Geometry check sheet. Reference: the model listing, model coordinates, mm. A direction names the side the tool comes from. Round coordinates to 2 decimals unless told otherwise and drop trailing zeros. Loops run counter-clockwise (first coordinate to the right, second up) from the corner with the lowest first, then second, coordinate; pieces in that order, holes last.
```python
from build123d import *

# Parameters (mm, degrees)
F0_R            = 6.35
F1_DEPTH        = 9.525
F2_W            = 9.5377
F2_H            = 31.75
F3_DEPTH        = 1.5875
F5_D            = 5.159375
F5_DEPTH        = 19.05
F5_TIP          = 1.5500326281
F7_D            = 3.571875
F7_DEPTH        = 19.05
F7_TIP          = 1.0730995118
F10_D           = 3.571875
F10_DEPTH       = 12.7
F10_TIP         = 1.0730995118
F10_ON_F9_D     = 3.571875
F10_ON_F9_DEPTH = 12.7
F10_ON_F9_TIP   = 1.0730995118


with BuildPart() as f1:
    # F0 (on Front) → F1 (new body)
    with BuildSketch(Plane.XZ):
        with BuildLine():
            Line((0, 50.8), (0, 0))
            Line((0, 0), (298.45, 0))
            Line((298.45, 0), (298.45, 50.8))
            Line((298.45, 50.8), (111.1377, 50.8))
            Line((111.1377, 50.8), (111.1377, 38.1))
            ThreePointArc((111.1377, 38.1), (114.3127, 34.925), (111.1377, 31.75))
            Line((111.1377, 31.75), (101.6, 31.75))
            ThreePointArc((101.6, 31.75), (98.425, 34.925), (101.6, 38.1))
            Line((101.6, 38.1), (101.6, 50.8))
            Line((101.6, 50.8), (88.9, 50.8))
            Line((88.9, 50.8), (88.9, 23.8125))
            ThreePointArc((88.9, 23.8125), (82.55, 17.4625), (76.2, 23.8125))
            Line((76.2, 23.8125), (76.2, 50.8))
            Line((76.2, 50.8), (0, 50.8))
        make_face()
        with Locations((250.19, 25.4)):
            Circle(F0_R, mode=Mode.SUBTRACT)
    extrude(amount=F1_DEPTH)

    # F2 (on face) → F3 (cut)
    with BuildSketch(Plane.XZ.offset(9.525)):
        with Locations((106.36885, 15.875)):
            Rectangle(F2_W, F2_H)
    extrude(amount=-F3_DEPTH, mode=Mode.SUBTRACT)

    # F5
    with Locations(Plane(origin=(0, 0, 0), x_dir=(0, -1, 0), z_dir=(-1, 0, 0))):
        with Locations((4.7625, 38.1), (4.7625, 25.4), (4.7625, 12.7)):
            Hole(F5_D / 2, depth=F5_DEPTH)
            with Locations((0, 0, -(F5_DEPTH + F5_TIP / 2))):  # 118° drill point
                Cone(0, F5_D / 2, F5_TIP, mode=Mode.SUBTRACT)

    # F7
    with Locations(Plane.XY.offset(31.75)):
        with Locations((106.36885, -3.96875)):
            Hole(F7_D / 2, depth=F7_DEPTH)
            with Locations((0, 0, -(F7_DEPTH + F7_TIP / 2))):  # 118° drill point
                Cone(0, F7_D / 2, F7_TIP, mode=Mode.SUBTRACT)

    # F10
    with Locations(Plane.XY.offset(50.8)):
        with Locations((38.1, -4.7625), (260.35, -4.7625)):
            Hole(F10_D / 2, depth=F10_DEPTH)
            with Locations((0, 0, -(F10_DEPTH + F10_TIP / 2))):  # 118° drill point
                Cone(0, F10_D / 2, F10_TIP, mode=Mode.SUBTRACT)

    # F10 on F9
    with Locations(Plane(origin=(0, 0, 0), x_dir=(1, 0, 0), z_dir=(0, 0, -1))):
        with Locations((260.35, 4.7625), (38.1, 4.7625)):
            Hole(F10_ON_F9_D / 2, depth=F10_ON_F9_DEPTH)
            with Locations((0, 0, -(F10_ON_F9_DEPTH + F10_ON_F9_TIP / 2))):  # 118° drill point
                Cone(0, F10_ON_F9_D / 2, F10_ON_F9_TIP, mode=Mode.SUBTRACT)


solid = f1.part
```
1) Mould release check, pull along Z, two halves, no side actions. Record for faces 1 (the face through (101.6, -5, 44)), 2 (the face through (39, -7, 50.8)), 3 (the face through (256.056, -4.696, 22.968)): +Z half, -Z half, draft (parallel to the pull), parting line (faces both ways), or undercut.
Report:
face 1: draft
face 2: +Z half
face 3: undercut
2) Scan lines: line 1 along X through (y, z) = (-7, 46); line 2 along Y through (x, z) = (260.35, 48) (3 decimals); line 3 along X through (y, z) = (-6, 21). Record each from-to range of solid material in increasing order.
Report:
line 1: x = 0 to 76.2, 88.9 to 101.6, 111.14 to 298.45
line 2: y = -9.525 to -6.548, -2.977 to 0
line 3: x = 0 to 76.86, 88.24 to 245.61, 254.77 to 298.45
3) Sectioned sample at B-B, the plane x = 82.55. Record the cut outline in (y, z) (1 decimal).
Report:
outline: (-9.5, 0) - (0, 0) - (0, 17.5) - (-9.5, 17.5) - close
4) Access from +Z, -Z, +X, -X, +Y, -Y to the whole of each face (thin tool, end or side, straight path). Record for faces 4 (the face through (9.658, -5.098, 40.658)), 5 (the face through (98.426, -4.696, 34.855)), 6 (the face through (88.9, -5, 37)).
Report:
face 4: -X
face 5: +Y, -Y
face 6: +Z, +Y, -Y
5) Sectioned sample at A-A, the plane x = 250.19. Record the cut outline in (y, z) (3 decimals), then the cut area to 3 significant figures.
Report:
outline: (-9.525, 0) - (0, 0) - (0, 19.05) - (-9.525, 19.05) - close; (-9.525, 31.75) - (0, 31.75) - (0, 50.8) - (-9.525, 50.8) - close
area: 363 mm2
6) Gauge pin test, flat ends, axial feed: pin 1 (5.5 mm diameter, centred on x = 260.35, y = -4.76, fed in from -Z); pin 2 (3 mm diameter, centred on x = 38.1, y = -4.76, fed in from +Z). Record the tip position at first contact, or that the pin passes through.
Report:
pin 1: stops at z = 0
pin 2: stops at z = 37.93
